Part model, mm, in its own coordinate system. A direction names the side the tool comes from. Round coordinates to 2 decimals unless told otherwise and drop trailing zeros. Write each loop counter-clockwise with the first axis right and the second up, starting at its lowest first coordinate (ties: lowest second). Pieces come first, ordered by that corner, then holes.
1) Pull direction Z, two halves, no side cores. Call faces 1 (the flat face through (4, 10, -4)), 2 (the flat face through (0, 0, 0)): +Z half, -Z half, draft (parallel to the pull), parting line (faces both ways), or undercut.
2) Saw through at D-D on y = 29.5. Write the cut outline in (x, z), and give its area (3 significant figures).
3) Which spindle directions (+Z, -Z, +X, -X, +Y, -Y) get a long thin tool onto all of the face, cutting with end or side? Do faces 3 (the flat face through (-5, 0, -10)), 4 (the flat face through (0, 5, 5.49)), 5 (the flat face through (-4, 10, 4)). Say none if no direction does.
4) Saw through at A-A on y = 4.5. Write the cut outline in (x, z) (1 decimal).
5) Saw through at B-B on z = 2. Write the cut outline in (x, y).
6) Saw through at C-C on x = 13.5. Write the cut outline in (y, z), and give its area (3 significant figures).
7) Flat gauge pins, fed straight in: pin 1 (4 mm diameter, centred on y = 29, z = -13.5, fed in from -X); pin 2 (4.5 mm diameter, centred on x = -4, z = 2.5, fed in from +Y); pin 3 (2.5 mm diameter, centred on y = 4, z = -0.5, fed in from -X). Where does each tip first touch, or does it go through?
8) Drill centre lines: L1, parallel to Z at x = 0, y = 10.5 (3 decimals); L2, parallel to Z at x = 0, y = 3; L3, parallel to X at y = 2.25, z = 0. Where is each one in solid material? Low to high.
```python
from build123d import *

# Parameters (mm, degrees)
SKETCH2_W           = 10.98
SKETCH2_H           = 10.98
BOSS_EXTRUDE1_DEPTH = 10
FILLET1_R           = 1


with BuildPart() as part:
    # Sketch2 → Boss-Extrude1 (new body)
    with BuildSketch(Plane(origin=(0, 0, 0), x_dir=(1, 0, 0), z_dir=(0, 1, 0))):
        Rectangle(SKETCH2_W, SKETCH2_H)
    extrude(amount=BOSS_EXTRUDE1_DEPTH)

    # Fillet1
    fillet1_edges = [part.edges().sort_by_distance(p)[0] for p in [
        (5.49, 5, 5.49),
        (-5.49, 5, 5.49),
        (-5.49, 5, -5.49),
        (5.49, 5, -5.49),
    ]]
    fillet(fillet1_edges, radius=FILLET1_R)

    # Sketch4 → Revolve1 (revolve)
    with BuildSketch(Plane(origin=(0, 0, 0), x_dir=(0, 0, -1), z_dir=(1, 0, 0))):
        with BuildLine():
            Line((22.912878475, 0), (11, 0))
            Line((11, 0), (11, 10))
            ThreePointArc((11, 10), (9.523392253, 15.504997729), (5.49, 19.53204595))
            Line((5.49, 19.53204595), (5.49, 10))
            Line((5.49, 10), (0, 10))
            Line((0, 10), (0, 35))
            ThreePointArc((0, 35), (20.916500663, 23.693063938), (22.912878475, 0))
        make_face()
    revolve(axis=Axis((0, 10, 0), (0, 1, 0)))


solid = part.part
```
Completed:
1. face 1: undercut
1. face 2: draft
2. outline: circle Ø31.29 at (0, 0)
2. area: 769 mm2
3. face 3: +Z, -Z, +X, -X, -Y
3. face 4: -Y
3. face 5: none
4. outline: circle Ø48.8 at (0, 0); (-5.5, -4.5) arc R1 ccw to (-4.5, -5.5) - (4.5, -5.5) arc R1 ccw to (5.5, -4.5) - (5.5, 4.5) arc R1 ccw to (4.5, 5.5) - (-4.5, 5.5) arc R1 ccw to (-5.5, 4.5) - close; hole circle Ø22 at (0, 0)
5. outline: (-22.83, 0) - (-10.82, 0) - (-10.82, 10) arc R10.82 cw to (-5.11, 19.53) - (-5.11, 10) - (-5.49, 10) - (-5.49, 0) - (5.49, 0) - (5.49, 10) - (5.11, 10) - (5.11, 19.53) arc R10.82 cw to (10.82, 10) - (10.82, 0) - (22.83, 0) arc R24.92 ccw (long way) to start
6. outline: (0, -18.51) arc R21.04 ccw (long way) to (0, 18.51) - close
6. area: 1,100 mm2
7. pin 1: stops at x = -13.08
7. pin 2: stops at y = 34.88
7. pin 3: stops at x = -24.54
8. L1: z = -24.995 to -10.989, -5.49 to 5.49, 10.989 to 24.995
8. L2: z = -24 to -11, -5.49 to 5.49, 11 to 24
8. L3: x = -23.77 to -11, -5.49 to 5.49, 11 to 23.77
